Solid Edge part; units mm, degrees
sketch "Sketch1" plane through (0, 0, 0) normal (0, 0, 1) x (1, 0, 0)
  line L0 (-33, -28) -> (33, -28)
  line L1 (33, -28) -> (33, 28)
  line L2 (33, 28) -> (-33, 28)
  line L3 (-33, 28) -> (-33, -28)
  dimension "D1" = 33
  dimension "D2" = 33
extrude "Protrusion1" add sketch "Sketch1" along normal blind 1
hole "Hole_1" at (-29, 24, 1) direction (0, 0, -1) diameter 3.2 end up to next
hole "Hole1" at (29, 24, 1) direction (0, 0, -1) diameter 3.2 end up to next
hole "Hole2" at (-29, -24, 1) direction (0, 0, -1) diameter 3.2 end up to next
hole "Hole3" at (29, -24, 1) direction (0, 0, -1) diameter 3.2 end up to next
properties material "Polyethylene, low density"
Work out the finished part from the listing and answer in its coordinate system (mm). Give positions to 0.01 mm unless a question says otherwise; leave off trailing zeros. Loops run counter-clockwise (first coordinate to the right, second up) from the corner with the lowest first, then second, coordinate; pieces in that order, holes last. Notation, with made-up numbers: M -26.5,24.5 L 26.5,24.5 A18 cw 26.5,29.5 Z; hole C 7,-2 d10. An arc over 180 degrees is marked long. One line per item, written item: value. Start each with the question number.
1. Each of these flat-tipped pins is pushed along its axis until it touches: P1, Ø3.5, axis at x = -29, y = -24, coming from the +Z side; P2, Ø2.5, axis at x = 29, y = -24, coming from the -Z side. Where does it stop, or does it pass through?
2. Find section A-A (x = -29). Give the vertices of the cut face in (y, z), and give its area (3 significant figures).
3. Find the intervals of material crossed by probe 1 along X at (y, z) = (-24, 0.45); probe 2 along Y at (x, z) = (29, 0.35); probe 3 along X at (y, z) = (23.5, 0.5), in increasing order.
4. Find section B-B (y = 24). Give the vertices of the cut face in (x, z).
5. Determine the mould class of faces 1 (the face through (0, 0, 1)), 2 (the face through (-27.414, -23.792, 0.507)), 3 (the face through (30.586, -23.792, 0.507)) for opening direction Y: released by +Y, released by -Y, zero draft, split by the parting line, or undercut.
Reported:
1. P1: stops at z = 1
1. P2: passes through
2. outline: M -28,0 L -25.6,0 L -25.6,1 L -28,1 Z; M -22.4,0 L 22.4,0 L 22.4,1 L -22.4,1 Z; M 25.6,0 L 28,0 L 28,1 L 25.6,1 Z
2. area: 49.6 mm²
3. probe 1: x = -33 to -30.6, -27.4 to 27.4, 30.6 to 33
3. probe 2: y = -28 to -25.6, -22.4 to 22.4, 25.6 to 28
3. probe 3: x = -33 to -30.52, -27.48 to 27.48, 30.52 to 33
4. outline: M -33,0 L -30.6,0 L -30.6,1 L -33,1 Z; M -27.4,0 L 27.4,0 L 27.4,1 L -27.4,1 Z; M 30.6,0 L 33,0 L 33,1 L 30.6,1 Z
5. face 1: zero draft
5. face 2: undercut
5. face 3: undercut
